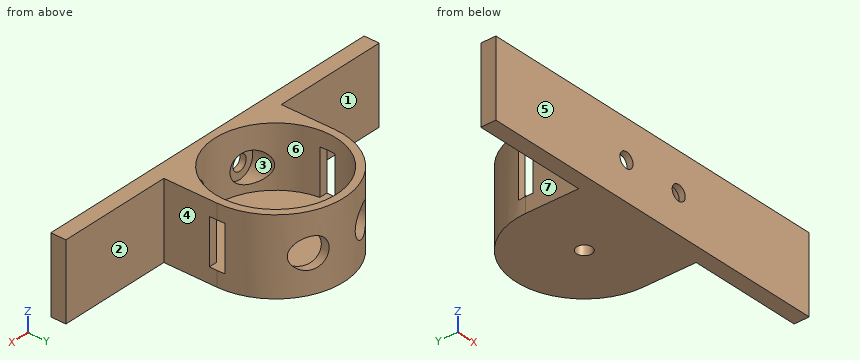
from build123d import *

# Parameters (mm, degrees)
SKETCH2_R           = 22.5
BOSS_EXTRUDE3_DEPTH = 25
SKETCH6_W           = 45
SKETCH6_H           = 22.5
BOSS_EXTRUDE4_DEPTH = 25
SKETCH4_R           = 20
CUT_EXTRUDE1_DEPTH  = 20
SKETCH5_R           = 2.5
CUT_EXTRUDE2_DEPTH  = 5
SKETCH7_R           = 5
CUT_EXTRUDE6_DEPTH  = 46
SKETCH9_R           = 5
SKETCH9_R_2         = 2.5
BOSS_EXTRUDE5_DEPTH = 2
SKETCH14_W          = 15
SKETCH14_H          = 5
CUT_EXTRUDE8_DEPTH  = 46.0000001
SKETCH15_W          = 25
SKETCH15_H          = 5
BOSS_EXTRUDE6_DEPTH = 37.5
SKETCH16_W          = 25
SKETCH16_H          = 5
BOSS_EXTRUDE7_DEPTH = 37.5


with BuildPart() as part:
    # Sketch2 → Boss-Extrude3 (new body)
    with BuildSketch(Plane.XY):
        Circle(SKETCH2_R)
    extrude(amount=BOSS_EXTRUDE3_DEPTH)

    # Sketch6 → Boss-Extrude4 (add)
    with BuildSketch(Plane.XY):
        with Locations((0, -11.25)):
            Rectangle(SKETCH6_W, SKETCH6_H)
    extrude(amount=BOSS_EXTRUDE4_DEPTH)

    # Sketch4 → Cut-Extrude1 (cut)
    with BuildSketch(Plane.XY.offset(25)):
        Circle(SKETCH4_R)
    extrude(amount=-CUT_EXTRUDE1_DEPTH, mode=Mode.SUBTRACT)

    # Sketch5 → Cut-Extrude2 (cut)
    with BuildSketch(Plane(origin=(0, 0, 0), x_dir=(-1, 0, 0), z_dir=(0, 0, -1))):
        Circle(SKETCH5_R)
    extrude(amount=-CUT_EXTRUDE2_DEPTH, mode=Mode.SUBTRACT)

    # Sketch7 → Cut-Extrude6 (cut, through all)
    with BuildSketch(Plane.XZ.offset(22.5)):
        with Locations((-10, 12.5)):
            Circle(SKETCH7_R)
        with Locations((10, 12.5)):
            Circle(SKETCH7_R)
    extrude(amount=-CUT_EXTRUDE6_DEPTH, mode=Mode.SUBTRACT)

    # Sketch9 → Boss-Extrude5 (add)
    with BuildSketch(Plane.XZ.offset(22.5)):
        with Locations((-10, 12.5)):
            Circle(SKETCH9_R)
        with Locations((-10, 12.5)):
            Circle(SKETCH9_R_2, mode=Mode.SUBTRACT)
        with Locations((10, 12.5)):
            Circle(SKETCH9_R)
        with Locations((10, 12.5)):
            Circle(SKETCH9_R_2, mode=Mode.SUBTRACT)
    extrude(amount=-BOSS_EXTRUDE5_DEPTH)

    # Sketch14 → Cut-Extrude8 (cut, through all)
    with BuildSketch(Plane(origin=(22.5, 0, 0), x_dir=(0, 0, -1), z_dir=(1, 0, 0))):
        with Locations((-12.5, 0)):
            Rectangle(SKETCH14_W, SKETCH14_H)
    extrude(amount=-CUT_EXTRUDE8_DEPTH, mode=Mode.SUBTRACT)

    # Sketch15 → Boss-Extrude6 (add)
    with BuildSketch(Plane.ZY.offset(22.5)):
        with Locations((12.5, -20)):
            Rectangle(SKETCH15_W, SKETCH15_H)
    extrude(amount=BOSS_EXTRUDE6_DEPTH)

    # Sketch16 → Boss-Extrude7 (add)
    with BuildSketch(Plane(origin=(22.5, 0, 0), x_dir=(0, 0, -1), z_dir=(1, 0, 0))):
        with Locations((-12.5, -20)):
            Rectangle(SKETCH16_W, SKETCH16_H)
    extrude(amount=BOSS_EXTRUDE7_DEPTH)


solid = part.part
The model under review builds one solid part; all positions refer to its coordinate system, in mm. Face numbers are marked on the shaded views. A direction names the side the tool comes from. Coordinates: 2 decimals unless noted, no trailing zeros. Loops run counter-clockwise (first coordinate to the right, second up) from the corner with the lowest first, then second, coordinate; pieces in that order, holes last. Notation, with made-up numbers: (1, 42.25) -> (21, 42.25) arc R24 ccw to (21, 69.25) -> close; hole circle Ø2 at (-18, -12.5). An arc over 180 degrees is marked (long way). Use a Markdown table: item, result. Add a question column.
1. Add section D-D on x = -28. Write out the cut boundary in (y, z), plus the area to 3 significant figures.
2. Add section C-C on y = -5.5. Write out the cut boundary in (x, z), plus the area to 3 significant figures.
3. To check wall thickness, follow line 1 (Y direction, x = 0, z = 13); line 2 (Y direction, x = 0, z = 3.65). State the ranges of each line that lie inside material, in increasing order.
4. Add section A-A on x = 0. Write out the cut boundary in (y, z), plus the area to 3 significant figures.
5. Clearance check with flat-ended pins moving along their axes: pin 1 Ø1.3 at (x, z) = (-21.5, 12) entering from +Y; pin 2 Ø6 at (x, y) = (0, 0) entering from +Z; pin 3 Ø8 at (x, z) = (-11, 10) entering from +Y; pin 4 Ø0.8 at (x, y) = (-21, -0.5) entering from -Z. State where each tip first meets the part, or that it passes through.
6. Add section B-B on z = 23. Write out the cut boundary in (x, y), plus the area to 3 significant figures.
7. Machinability: for the marked faces 1, 2 and 3, which of the approach directions +Z, -Z, +X, -X, +Y, -Y give a long, thin tool a straight path to every point of the face, cutting with its end or side? Answer none if there is none.
8. Draft analysis for pull direction X (two halves, no side actions). For the marked faces 4, 5, 6 and 7, state which applies: pulls with the +X half, pulls with the -X half, needs draft (parallel to the pull), parting line crosses it, or undercut.
Returned:
| question | item | result |
|---|---|---|
| 1 | outline | (-22.5, 0) -> (-17.5, 0) -> (-17.5, 25) -> (-22.5, 25) -> close |
| 1 | area | 125 mm² |
| 2 | outline | (-22.5, 0) -> (22.5, 0) -> (22.5, 25) -> (19.23, 25) -> (19.23, 5) -> (-19.23, 5) -> (-19.23, 25) -> (-22.5, 25) -> close |
| 2 | area | 356 mm² |
| 3 | line 1 | y = -22.5 to -20, 20 to 22.5 |
| 3 | line 2 | y = -22.5 to -2.5, 2.5 to 22.5 |
| 4 | outline | (-22.5, 0) -> (-2.5, 0) -> (-2.5, 5) -> (-20, 5) -> (-20, 25) -> (-22.5, 25) -> close; (2.5, 0) -> (22.5, 0) -> (22.5, 25) -> (20, 25) -> (20, 5) -> (2.5, 5) -> close |
| 4 | area | 300 mm² |
| 5 | pin 1 | stops at y = 8.46 |
| 5 | pin 2 | stops at z = 5 |
| 5 | pin 3 | stops at y = 21.24 |
| 5 | pin 4 | stops at z = 0 |
| 6 | outline | (-60, -22.5) -> (60, -22.5) -> (60, -17.5) -> (22.5, -17.5) -> (22.5, 0) arc R22.5 ccw to (-22.5, 0) -> (-22.5, -17.5) -> (-60, -17.5) -> close; hole circle Ø40 at (0, 0) |
| 6 | area | 926 mm² |
| 7 | face 1 | +Z, -Z, -X, +Y |
| 7 | face 2 | +Z, -Z, +X, +Y |
| 7 | face 3 | +Y |
| 8 | face 4 | pulls with the +X half |
| 8 | face 5 | needs draft |
| 8 | face 6 | undercut |
| 8 | face 7 | pulls with the -X half |
